```python
from build123d import *

# Parameters (mm, degrees)
SKETCH1_R                = 7.5
SKETCH1_R_2              = 3
BOSS_EXTRUDE1_DEPTH      = 9
BOSS_EXTRUDE2_REACH      = 112.622
BOSS_EXTRUDE2_END_RADIUS = 7.5
BOSS_EXTRUDE3_REACH      = 207.334
BOSS_EXTRUDE3_END_RADIUS = 7.5
FILLET1_START            = -7.245522841
FILLET1_DEPTH            = 14.745522841


with BuildPart() as part:
    # Sketch1 → Boss-Extrude1 (new body)
    with BuildSketch(Plane(origin=(0, 0, 0), x_dir=(1, 0, 0), z_dir=(0, 1, 0))):
        with Locations(Location((0, 0, 0), (0, 0, 270))):
            Circle(SKETCH1_R)
        with Locations(Location((0, 0, 0), (0, 0, 270))):
            Circle(SKETCH1_R_2, mode=Mode.SUBTRACT)
    extrude(amount=BOSS_EXTRUDE1_DEPTH)

    # Boss-Extrude2: up to this cylinder (the profile starts outside it)
    boss_extrude2_end = Plane(origin=(0, 4.5, 0), z_dir=(0, -1, 0)) * Cylinder(BOSS_EXTRUDE2_END_RADIUS, 241.244, mode=Mode.PRIVATE)
    # Sketch3 → Boss-Extrude2 (add, up to the surface)
    with BuildSketch(Plane(origin=(102.5, 0, 0), x_dir=(0, 0, -1), z_dir=(1, 0, 0)), mode=Mode.PRIVATE) as boss_extrude2_sk1:
        Polygon((-6, 9), (7.245522841, 0), (6, 0), (-7.245522841, 9), align=None)
    boss_extrude2_tool1 = extrude(boss_extrude2_sk1.sketch, amount=-BOSS_EXTRUDE2_REACH, mode=Mode.PRIVATE) - boss_extrude2_end
    add(boss_extrude2_tool1.solids().sort_by_distance((102.5, 4.5, 0))[0])

    # Boss-Extrude3: up to this cylinder (the profile starts outside it)
    boss_extrude3_end = Plane(origin=(0, 4.5, 0), z_dir=(0, -1, 0)) * Cylinder(BOSS_EXTRUDE3_END_RADIUS, 430.668, mode=Mode.PRIVATE)
    # Sketch5 → Boss-Extrude3 (add, up to the surface)
    with BuildSketch(Plane(origin=(-102.5, 0, 0), x_dir=(0, 0, -1), z_dir=(1, 0, 0)), mode=Mode.PRIVATE) as boss_extrude3_sk1:
        Polygon((5.784000547, 9), (-7, 0), (-5.784000547, 0), (7, 9), align=None)
    boss_extrude3_tool1 = extrude(boss_extrude3_sk1.sketch, amount=BOSS_EXTRUDE3_REACH, mode=Mode.PRIVATE) - boss_extrude3_end
    add(boss_extrude3_tool1.solids().sort_by_distance((-102.5, 4.5, 0))[0])

    # Fillet1: read off the stored shape, not the designer's step
    # Fillet1 outline → Fillet1 (cut)
    with BuildSketch(Plane.XY.offset(FILLET1_START)):
        with BuildLine():
            ThreePointArc((-102.5, 0), (-95.283539892, 6.606816862), (-85.796706912, 9))
            Line((-85.796706912, 9), (-102.5, 9))
            Line((-102.5, 9), (-102.5, 0))
        make_face()
        with BuildLine():
            ThreePointArc((85.796706911, 9), (95.283539892, 6.606816862), (102.5, 0))
            Line((102.5, 0), (102.5, 9))
            Line((102.5, 9), (85.796706911, 9))
        make_face()
    extrude(amount=FILLET1_DEPTH, mode=Mode.SUBTRACT)


solid = part.part
```
Could you check a few things on this model? Use its own coordinates, in mm. A direction names the side the tool comes from. Coordinates: 2 decimals unless noted, no trailing zeros. Loops run counter-clockwise (first coordinate to the right, second up) from the corner with the lowest first, then second, coordinate; pieces in that order, holes last.
1) Imagine slicing it at C-C (z = 0). List the corners of the cut face in (x, y) for me.
Reported:
outline: (-98.94, 4.07) - (-7.5, 4.07) - (-7.5, 0) - (-3, 0) - (-3, 9) - (-7.5, 9) - (-7.5, 4.93) - (-97.89, 4.93) arc R20 ccw to start; (3, 0) - (7.5, 0) - (7.5, 4.08) - (98.94, 4.08) arc R20 ccw to (97.9, 4.92) - (7.5, 4.92) - (7.5, 9) - (3, 9) - close
2) Imagine slicing it at B-B (y = 4.5). List the corners of the cut face in (x, z) for me, and give its area (3 significant figures).
Reported:
outline: (-98.44, -0.61) - (-7.48, -0.61) arc R7.5 ccw to (7.47, -0.62) - (98.44, -0.62) - (98.44, 0.62) - (7.47, 0.62) arc R7.5 ccw to (-7.48, 0.61) - (-98.44, 0.61) - close; hole circle Ø6 at (0, 0)
area: 372 mm2
3) Which directions (+Z, -Z, +X, -X, +Y, -Y) give clear straight access to the entire face, cutting with the end or side of a thin tool? Please do faces 1 (the face through (-0.1, 4.4, 7.5)), 2 (the face through (0.5, 0, -3.4)).
Reported:
face 1: none
face 2: +Z, -Z, +X, -X, -Y
4) Thinking about a two-plate mould opening in X: for faces 3 (the face through (0.9, 4.44, 2.86)), 4 (the face through (-96, 6.2, -2.1)), 5 (the face through (7, 9, 1)), 6 (the face through (95.88, 6.27, 2.65)), which applies, released by +X, released by -X, zero draft, split by the parting line, or undercut?
Reported:
face 3: undercut
face 4: released by -X
face 5: zero draft
face 6: released by +X
5) Imagine slicing it at A-A (x = 0). List the corners of the cut face in (y, z) for me, and give its area (3 significant figures).
Reported:
outline: (0, -7.5) - (9, -7.5) - (9, -3) - (0, -3) - close; (0, 3) - (9, 3) - (9, 7.5) - (0, 7.5) - close
area: 81.0 mm2
6) Please list where these lines run through material, in increasing order: line 1 along X through (y, z) = (3, 0); line 2 along X through (y, z) = (1, -1.25); line 3 along Z through (x, y) = (1, 6.75).
Reported:
line 1: x = -7.5 to -3, 3 to 7.5
line 2: x = -7.4 to -2.73, 2.73 to 7.4
line 3: z = -7.43 to -2.83, 2.83 to 7.43
7) Will these pins go through, and if not, where does the flat tip stop? pin 1 Ø5 at (x, z) = (-78.5, 2.5) entering from +Y; pin 2 Ø3 at (x, y) = (-61, 3.5) entering from -Z; pin 3 Ø6 at (x, z) = (-40.5, -0.5) entering from +Y.
Reported:
pin 1: stops at y = 4.93
pin 2: stops at z = -1.32
pin 3: stops at y = 7.39
8) Imagine slicing it at D-D (x = 22). List the corners of the cut face in (y, z) for me.
Reported:
outline: (0, -7.25) - (9, 6) - (9, 7.25) - (0, -6) - close
